from build123d import *

# Parameters (mm, degrees)
SKETCH1_R           = 35
SKETCH1_R_2         = 7.5
SKETCH1_R_3         = 3
BOSS_EXTRUDE1_DEPTH = 2
CHAMFER1_SIZE       = 1.6


with BuildPart() as part:
    # Sketch1 → Boss-Extrude1 (new body)
    with BuildSketch(Plane.XY):
        Circle(SKETCH1_R)
        Circle(SKETCH1_R_2, mode=Mode.SUBTRACT)
        with Locations((25, 0)):
            Circle(SKETCH1_R_3, mode=Mode.SUBTRACT)
        with Locations((0, -25)):
            Circle(SKETCH1_R_3, mode=Mode.SUBTRACT)
        with Locations((-25, 0)):
            Circle(SKETCH1_R_3, mode=Mode.SUBTRACT)
        with Locations((0, 25)):
            Circle(SKETCH1_R_3, mode=Mode.SUBTRACT)
    extrude(amount=BOSS_EXTRUDE1_DEPTH)

    # Chamfer1
    chamfer1_edges = [part.edges().sort_by_distance(p)[0] for p in [
        (-35, 0, 0),
    ]]
    chamfer(chamfer1_edges, length=CHAMFER1_SIZE)


solid = part.part
Read the model definition and answer for the solid it produces. Units are mm, in the model's axes. Coordinates: 2 decimals unless noted, no trailing zeros. Write each loop counter-clockwise with the first axis right and the second up, starting at its lowest first coordinate (ties: lowest second). Pieces come first, ordered by that corner, then holes. Notation, with made-up numbers: (9.5, 3) -> (15.5, 3) arc R15 cw to (15.5, 28) -> close; hole circle Ø9 at (34, -7.5). An arc over 180 degrees is marked (long way). Return JSON: item names as keys, results as strings.
(1) For a pull along X with two mould halves and no side action, classify faces 1 (the cylindrical face through (-7.493, 0.33, 0.986)), 2 (the flat face through (0, 8, 2)), 3 (the cylindrical face through (-27.77, -21.3, 1.8)), 4 (the cylindrical face through (22, 0, 1)) as pulls with the +X half, pulls with the -X half, needs draft (parallel to the pull), parting line crosses it, or undercut.
Answers below:
{"face 1": "undercut", "face 2": "needs draft", "face 3": "parting line crosses it", "face 4": "undercut"}
(2) Consider line 1 along X through (y, z) = (0.5, 0.2); line 2 along X through (y, z) = (-23.5, 1.2); line 3 along Y through (x, z) = (0, 1.4). Determine where each line is inside the solid, lowest interval first. Write a range as from..to.
Answers below:
{"line 1": "-33.6..-27.96, -22.04..-7.48, 7.48..22.04, 27.96..33.6", "line 2": "-25.4..-2.6, 2.6..25.4", "line 3": "-34.8..-28, -22..-7.5, 7.5..22, 28..34.8"}
(3) The part is cut by section C-C on y = 1.5. State how many separate pieces and enclosed holes the cut face has, then the cut area to 3 significant figures.
Answers below:
{"separate pieces": "4", "enclosed holes": "0", "area": "87.1 mm^2"}
(4) The part is cut by section A-A on x = 0. Give the vertices of the cut face in (y, z).
Answers below:
{"outline": "(-35, 1.6) -> (-33.4, 0) -> (-28, 0) -> (-28, 2) -> (-35, 2) -> close; (-22, 0) -> (-7.5, 0) -> (-7.5, 2) -> (-22, 2) -> close; (7.5, 0) -> (22, 0) -> (22, 2) -> (7.5, 2) -> close; (28, 0) -> (33.4, 0) -> (35, 1.6) -> (35, 2) -> (28, 2) -> close"}
(5) The part is cut by section B-B on z = 1.1. Give the vertices of the cut face in (x, y).
Answers below:
{"outline": "circle Ø69 at (0, 0); hole circle Ø6 at (-25, 0); hole circle Ø15 at (0, 0); hole circle Ø6 at (0, -25); hole circle Ø6 at (0, 25); hole circle Ø6 at (25, 0)"}
